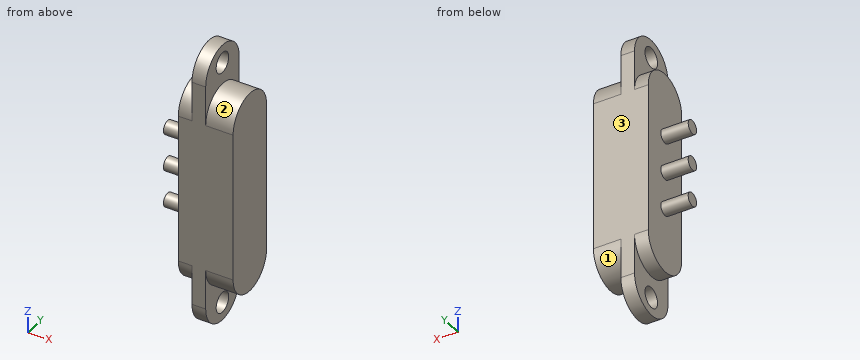
Autodesk Inventor part; units mm, degrees
ref_plane "YZ Plane" through (0, 0, 0) normal (1, 0, 0) x (0, 1, 0)
ref_plane "XZ Plane" through (0, 0, 0) normal (0, 1, 0) x (-1, 0, 0)
ref_plane "XY Plane" through (0, 0, 0) normal (0, 0, 1) x (1, 0, 0)
sketch "Sketch1" plane through (0, 0, 0) normal (0, 1, 0) x (-1, 0, 0)
  line L0 (-2, 7.5) -> (2, 7.5)
  line L1 (2, 7.5) -> (2, -7.5)
  line L2 (2, -7.5) -> (-2, -7.5)
  line L3 (-2, -7.5) -> (-2, 7.5)
  line L4 (-2, 7.5) -> (2, -7.5) construction
  line L5 (2, 7.5) -> (-2, -7.5) construction
  point P0 (0, 0)
  dimension "d0" = 4
  dimension "d1" = 15
extrude "Extrusion1" add sketch "Sketch1" along normal blind 4
sketch "Sketch2" plane through (2, 0, 7.5) normal (1, 0, 0) x (0, 0, -1)
  line L0 (0, 0) -> (0, 4)
  line L1 (0, 2) -> (15, 2) construction
  line L2 (15, 0) -> (15, 4)
  line L3 (2, 0) -> (13, 0)
  line L4 (13, 4) -> (2, 4)
  arc A0 (2, 4) -> (2, 0) centre (2, 2) ccw
  arc A1 (13, 0) -> (13, 4) centre (13, 2) ccw
  line L5 (0, 4) -> (15, 4)
  line L6 (0, 0) -> (15, 0)
  point P0 (7.5, 0)
  point P1 (7.5, 2)
  point P2 (15, 2)
extrude "Extrusion2" cut sketch "Sketch2" against normal blind 2 contours L0 A0 L6 | L0 L5 A0 | A1 L2 L6 | L5 L2 A1
sketch "Sketch3" plane through (-2, 0, -7.5) normal (-1, 0, 0) x (0, 0, 1)
  arc A0 (2, 4) -> (0, 2) centre (2, 2) ccw
  line L0 (0, 0) -> (0, 4)
  line L1 (0, 4) -> (15, 4)
  arc A1 (0, 2) -> (2, 0) centre (2, 2) ccw
  arc A2 (2, 4) -> (2, 0) centre (2, 2) ccw
  line L2 (13, 4) -> (2, 4)
  arc A3 (13, 0) -> (13, 4) centre (13, 2) ccw
  line L3 (13, 0) -> (2, 0)
  line L4 (15, 0) -> (15, 4)
  line L5 (0, 0) -> (15, 0)
  point P0 (7.5, 0)
  point P1 (15, 2)
extrude "Extrusion3" cut sketch "Sketch3" against normal blind 1 contours A0 L0 L1 | A1 L5 L0 | L1 L4 A3 | L4 L5 A3
sketch "Sketch4" plane through (-2, 0, -5.5) normal (-1, 0, 0) x (0, 0, 1)
  arc A0 (0, 4) -> (-2, 2) centre (0, 2) ccw
  circle A1 centre (0, 2) radius 1.5
  arc A2 (13, 2) -> (11, 4) centre (11, 2) ccw
  circle A3 centre (11, 2) radius 1.5
  point P0 (5.5, 0)
  dimension "d8" = 3
  dimension "d9" = 3
mark "Mark1"
sketch "Sketch5" plane through (-2, 0, -5.5) normal (-1, 0, 0) x (0, 0, 1)
  circle A0 centre (2.75, 2) radius 1
  circle A1 centre (0, 2) radius 1.5
  circle A2 centre (11, 2) radius 1.5
  line L0 (0, 4) -> (11, 4)
  circle A3 centre (5.5, 2) radius 1
  circle A4 centre (8.25, 2) radius 1
  point P0 (5.5, 0)
  dimension "d10" = 2
  dimension "d11" = 2.75
  dimension "d12" = 11
  dimension "d15" = 2.75
mark "Mark2"
sketch "Sketch6" plane through (-2, 2, -2.75) normal (-1, 0, 0) x (0, 0, 1)
  circle A0 centre (0, 0) radius 1
  circle A1 centre (0, 0) radius 0.5
  circle A2 centre (2.75, 0) radius 1
  circle A3 centre (2.75, 0) radius 0.5
  circle A4 centre (5.5, 0) radius 1
  circle A5 centre (5.5, 0) radius 0.5
  point P0 (2.75, -2)
  dimension "d20" = 1
  dimension "d21" = 1
  dimension "d38" = 1
extrude "Extrusion4" add sketch "Sketch6" along normal blind 2 contours A1 | A3 | A5
sketch "Sketch7" plane through (2, 0, 5.5) normal (1, 0, 0) x (0, 0, -1)
  circle A0 centre (0, 2) radius 1.5
  circle A1 centre (11, 2) radius 1.5
  point P0 (5.5, 0)
mark "Mark3"
sketch "Sketch8" plane through (2, 0, 5.5) normal (1, 0, 0) x (0, 0, -1)
  circle A0 centre (8.25, 2) radius 1
  circle A1 centre (5.5, 2) radius 1
  circle A2 centre (5.5, 2) radius 0.75
  circle A3 centre (8.25, 2) radius 0.75
  circle A4 centre (2.75, 2) radius 1
  circle A5 centre (2.75, 2) radius 0.75
  point P0 (5.5, 0)
  dimension "d24" = 1.5
  dimension "d25" = 1.5
  dimension "d39" = 1.5
mark "Mark4"
sketch "Sketch11" plane through (0, 0, 7.5) normal (1, 0, 0) x (0, 0, -1)
  line L0 (-2.93, 2) -> (17.93, 2) construction
  line L1 (-0.93, 0) -> (15.93, 0)
  line L2 (15.93, 4) -> (-0.93, 4)
  arc A0 (-0.93, 4) -> (-0.93, 0) centre (-0.93, 2) ccw
  arc A1 (15.93, 0) -> (15.93, 4) centre (15.93, 2) ccw
  line L3 (2, 0) -> (13, 0)
  point P0 (7.5, 0)
  point P1 (7.5, 2)
  point P2 (7.5, 4)
  point P3 (7.5, 0)
  dimension "d31" = 20.86
extrude "Extrusion7" add sketch "Sketch11" against normal blind 1
sketch "Sketch12" plane through (0, 0, 7.5) normal (1, 0, 0) x (0, 0, -1)
  arc A0 (-0.93, 4) -> (-0.93, 0) centre (-0.93, 2) ccw
  circle A1 centre (-1.6, 2) radius 0.75
  circle A2 centre (2, 2) radius 1.5
  point P0 (7.5, 0)
  dimension "d34" = 1.5
  dimension "d35" = 3.6
extrude "Extrusion8" cut sketch "Sketch12" against normal blind 1 contours A1
mirror "Mirror1" about plane through (0, 0, 0) normal (0, 0, 1) of "Extrusion8"
equation "\"d9\" = d8"
equation "\"d11\" = 0.25 * d12"
equation "\"d15\" = d11"
equation "\"d21\" = d20"
equation "\"d38\" = d21"
equation "\"d25\" = d24"
equation "\"d39\" = d24"
properties part number "3_pin_ear_female"
Model file for the job. Use its own axes, mm. Face numbers are marked on the shaded views. A direction names the side the tool comes from. Round coordinates to 2 decimals unless told otherwise and drop trailing zeros. Loops run counter-clockwise (first coordinate to the right, second up) from the corner with the lowest first, then second, coordinate; pieces in that order, holes last. Notation, with made-up numbers: M -23,56 L -6,56 A23 ccw -6,77 Z; hole C -24.75,-5.5 d10. An arc over 180 degrees is marked long. Put each result on its own line as item: value. Start each with the question number.
Item 1: 3-axis set-ups, long thin cutter, end or side, ignore diameter. For the marked faces 1, 2 and 3: which of +Z, -Z, +X, -X, +Y, -Y reach the whole face in a straight line?
Item 2: Cut at D-D (y = 1). List the corners of the cut face in (x, z).
Item 3: Cut at B-B (z = -2.75). List the corners of the cut face in (x, y).
Item 4: Cut at C-C (z = -9.1). List the corners of the cut face in (x, y).
Item 5: Cut at A-A (y = 2). Give the number of separate pieces and of enclosed holes in the cut face, then the cut area to 3 significant figures.
Item 6: Drop flat-ended pins along their axis: P1, Ø0.9, axis at y = 2, z = -9.1, coming from the -X side; P2, Ø1.7, axis at y = 2, z = 9.1, coming from the -X side; P3, Ø2, axis at y = 1.5, z = 8, coming from the -X side; P4, Ø2, axis at x = 0, y = 0.5, coming from the -Z side. Give the stop position or say it passes through.
Item 7: Drill centre lines: line 1 along Z through (x, y) = (-2.9, 1.8); line 2 along X through (y, z) = (1.9, 1.5); line 3 along Z through (x, y) = (-3.6, 1.7). Where is each one in solid material? Low to high.
Answer block:
1. face 1: -Z, +X
1. face 2: +Z, +X
1. face 3: +Z, -Z, +X, -X, +Y
2. outline: M -2,-7.23 L -1,-7.23 L -1,-10.16 L 0,-10.16 L 0,-7.23 L 2,-7.23 L 2,7.23 L 0,7.23 L 0,10.16 L -1,10.16 L -1,7.23 L -2,7.23 Z
3. outline: M -4,1.5 L -2,1.5 L -2,0 L 2,0 L 2,4 L -2,4 L -2,2.5 L -4,2.5 Z
4. outline: M -1,0.12 L 0,0.12 L 0,1.25 L -1,1.25 Z; M -1,2.75 L 0,2.75 L 0,3.88 L -1,3.88 Z
5. separate pieces: 3
5. enclosed holes: 0
5. area: 68.9 mm2
6. P1: through
6. P2: x = -1
6. P3: x = -2
6. P4: z = -10.37
7. line 1: -3.21 to -2.29, -0.46 to 0.46, 2.29 to 3.21
7. line 2: -2 to 2
7. line 3: -3.15 to -2.35, -0.4 to 0.4, 2.35 to 3.15
